Work out the finished part from the listing and answer in its coordinate system (mm). Give positions to 0.01 mm unless a question says otherwise; leave off trailing zeros. Order: outer loops, then holes, each group sorted by start corner. A loop starts at its lowest first (then second) coordinate and runs counter-clockwise, first axis right, second up. Notation, with made-up numbers: (57.5, -19) - (67.5, -19) arc R34 cw to (67.5, 11) - close; hole circle Ø10 at (12, 23). An arc over 180 degrees is marked (long way). Put each result on its own line as item: value.
```python
from build123d import *

# Parameters (mm, degrees)
F0_W     = 60
F0_H     = 97.64
F0_R     = 1.7
F1_DEPTH = 23
F3_D     = 6
F3_DEPTH = 8
F3_TIP   = 1.8025818571
F2_W     = 10.5
F2_H     = 6.3
F4_DEPTH = 4.75
F2_W_2   = 15.13
F2_H_2   = 10.44
F5_DEPTH = 1.75


with BuildPart() as f1:
    # F0 (on Front) → F1 (new body)
    with BuildSketch(Plane.XZ):
        with Locations((0.968804583, 14.7747536898)):
            Rectangle(F0_W, F0_H)
        with Locations((18.098804583, 49.1747536898)):
            Circle(F0_R, mode=Mode.SUBTRACT)
    extrude(amount=F1_DEPTH)

    # F3
    with Locations(Plane.XY.offset(63.5947536898)):
        with Locations((5.268804583, -14)):
            Hole(F3_D / 2, depth=F3_DEPTH)
            with Locations((0, 0, -(F3_DEPTH + F3_TIP / 2))):  # 118° drill point
                Cone(0, F3_D / 2, F3_TIP, mode=Mode.SUBTRACT)

    # F2 (on face) → F4 (join)
    with BuildSketch(Plane.XY.offset(63.5947536898)):
        with Locations((-15.0949036926, -15.4)):
            Rectangle(F2_W, F2_H)
    extrude(amount=F4_DEPTH)

    # F2 (on face) → F5 (join)
    with BuildSketch(Plane.XY.offset(63.5947536898)):
        with Locations((-14.9943149662, -15.38)):
            Rectangle(F2_W_2, F2_H_2)
        with Locations((-15.0949036926, -15.4)):
            Rectangle(F2_W, F2_H, mode=Mode.SUBTRACT)
    extrude(amount=F5_DEPTH)


solid = f1.part
```
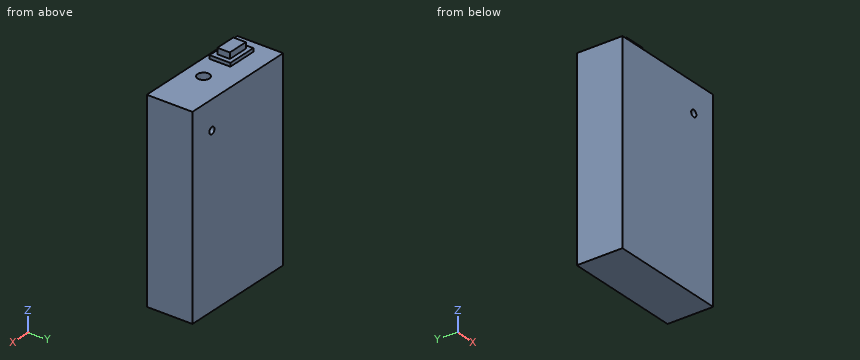
(1) Straight lines are drawn through the part: line 1 (X direction, y = -14, z = 61.25); line 2 (Z direction, x = -13.5, y = -8.5); line 3 (Z direction, x = -8, y = -13). For each, find the intervals that lie inside material, in ascending order.
Geometry check:
line 1: x = -29.03 to 2.27, 8.27 to 30.97
line 2: z = -34.05 to 63.59
line 3: z = -34.05 to 65.34
(2) Section B-B, the plane y = -8.75 is taken. Write down the section's boundary in (x, z).
Geometry check:
outline: (-29.03, -34.05) - (30.97, -34.05) - (30.97, 63.59) - (-29.03, 63.59) - close; hole circle Ø3.4 at (18.1, 49.17)
(3) Section A-A, the plane x = 15 is taken. Write down the section's boundary in (y, z), then the cut area to 3 significant figures.
Geometry check:
outline: (-23, -34.05) - (0, -34.05) - (0, 63.59) - (-23, 63.59) - close
area: 2,250 mm²
(4) Given pin 1 (1.9 mm diameter, centred on y = -14, z = 65, fed in from -X); pin 2 (0.5 mm diameter, centred on x = -16.5, z = 64.5, fed in from -Y); pin 3 (8 mm diameter, centred on x = 22.5, y = -16, fed in from +Z), each flat-ended and moving along its own axis, determine where each tip first touches the part or whether it passes through.
Geometry check:
pin 1: stops at x = -22.56
pin 2: stops at y = -20.6
pin 3: stops at z = 63.59
